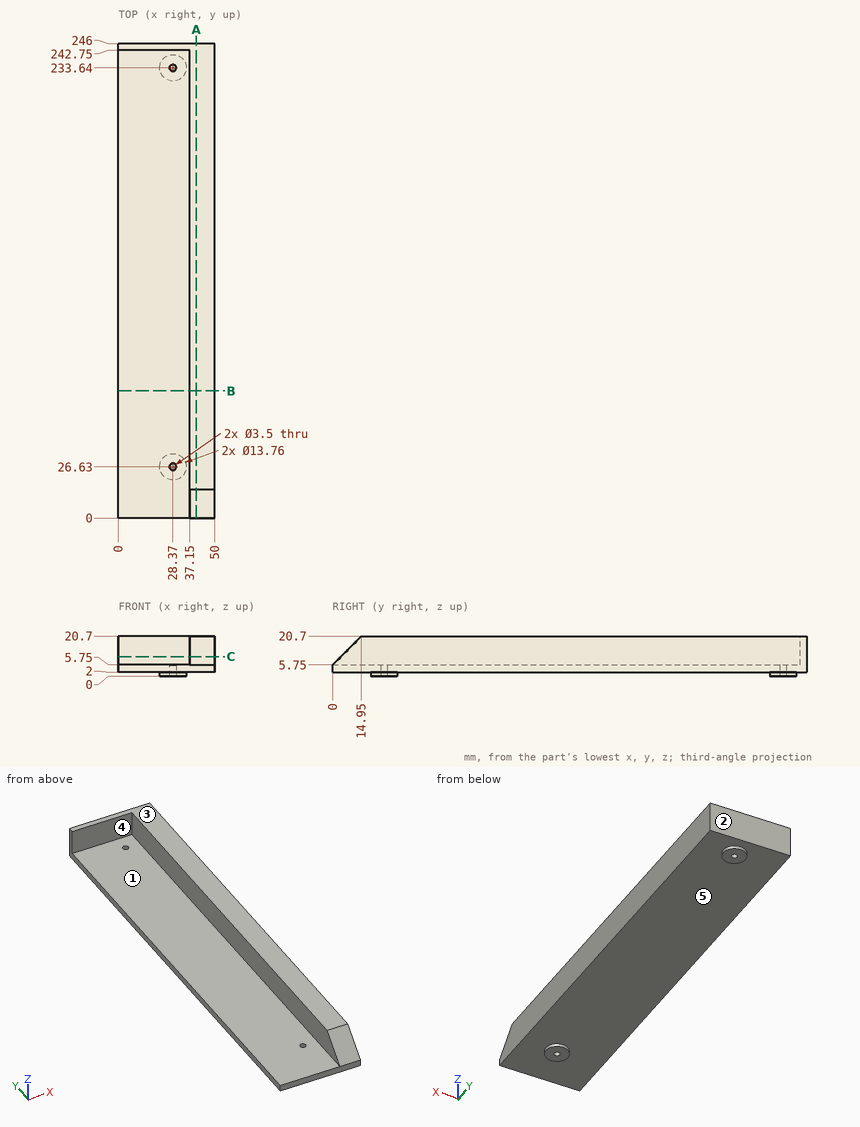
Here's the drawing with two shaded views (mm, measured from the low corner). I have some questions. A direction names the side the tool comes from. Give positions to 0.01 mm unless a question says otherwise; leave off trailing zeros. Loops run counter-clockwise (first coordinate to the right, second up) from the corner with the lowest first, then second, coordinate; pieces in that order, holes last. Notation, with made-up numbers: M 7.25,16.5 L 41.25,16.5 A27 cw 41.25,35.5 Z; hole C -0.75,-27 d1. An arc over 180 degrees is marked long. One line per item, written item: value.
1) Imagine slicing it at C-C on z = 10. Write out the boundary of the cut face in (x, y), and give its area (3 significant figures).
Geometry check:
outline: M 0,242.75 L 37.15,242.75 L 37.15,4.25 L 50,4.25 L 50,246 L 0,246 Z
area: 3,230 mm²
2) Imagine slicing it at B-B on y = 66. Write out the boundary of the cut face in (x, z).
Geometry check:
outline: M 0,2 L 50,2 L 50,20.7 L 37.15,20.7 L 37.15,5.75 L 0,5.75 Z
3) Thinking about a two-plate mould opening in Y: for the marked faces 3, 4 and 5, which applies, +Y half, -Y half, draft (parallel to the pull), parting line (faces both ways), or undercut?
Geometry check:
face 3: draft
face 4: -Y half
face 5: undercut
4) I'm going to push flat-ended pins straight in: pin 1 (12 mm diameter, centred on x = 24.5, y = 178.5, fed in from -Z); pin 2 (2 mm diameter, centred on y = 126, z = 10.5, fed in from -X); pin 3 (4 mm diameter, centred on x = 28.37, y = 233.64, fed in from +Z). Where does each tip first touch, or does it pass through?
Geometry check:
pin 1: stops at z = 2
pin 2: stops at x = 37.15
pin 3: stops at z = 5.75
5) Please list where these lines run through material, in increasing order: line 1 (Y direction, x = 28.37, z = 3.45); line 2 (X direction, y = 233.64, z = 3.9); line 3 (Z direction, x = 43.5, y = 64).
Geometry check:
line 1: y = 0 to 24.88, 28.38 to 231.89, 235.39 to 246
line 2: x = 0 to 26.62, 30.12 to 50
line 3: z = 2 to 20.7
6) On a 3-axis mill with a long thin cutter (end or side, diameter ignored), from which of +Z, -Z, +X, -X, +Y, -Y can I reach the whole of each face in a straight line? I mean the marked faces 1 and 2. Say none if no direction works.
Geometry check:
face 1: +Z, -X, -Y
face 2: +Z, -Z, +X, -X, +Y
7) Imagine slicing it at A-A on x = 40.5. Write out the boundary of the cut face in (y, z).
Geometry check:
outline: M 0,2 L 246,2 L 246,20.7 L 14.95,20.7 L 0,5.75 Z
